from build123d import *

# Parameters (mm, degrees)
SKETCH1_W           = 113
SKETCH1_H           = 53
SKETCH1_R           = 1.25
BOSS_EXTRUDE1_DEPTH = 1.8
SKETCH2_W           = 17
SKETCH2_H           = 12
SKETCH2_W_2         = 8
SKETCH2_H_2         = 14
SKETCH2_W_3         = 18
SKETCH2_H_3         = 10
BOSS_EXTRUDE2_DEPTH = 11


with BuildPart() as part:
    # Sketch1 → Boss-Extrude1 (new body)
    with BuildSketch(Plane.XY):
        with Locations((-56.5, 26.5)):
            Rectangle(SKETCH1_W, SKETCH1_H)
        with Locations((-3, 3)):
            Circle(SKETCH1_R, mode=Mode.SUBTRACT)
        with Locations((-3, 50)):
            Circle(SKETCH1_R, mode=Mode.SUBTRACT)
        with Locations((-105, 50)):
            Circle(SKETCH1_R, mode=Mode.SUBTRACT)
        with Locations((-105, 3)):
            Circle(SKETCH1_R, mode=Mode.SUBTRACT)
    extrude(amount=BOSS_EXTRUDE1_DEPTH)

    # Sketch2 → Boss-Extrude2 (add)
    with BuildSketch(Plane.XY.offset(1.8)):
        with Locations((-9.223845793, 31)):
            Rectangle(SKETCH2_W, SKETCH2_H)
        with Locations((-23.223845793, 42)):
            Rectangle(SKETCH2_W_2, SKETCH2_H_2)
        with Locations((-104, 40)):
            Rectangle(SKETCH2_W_3, SKETCH2_H_3)
        with Locations((-104, 13)):
            Rectangle(SKETCH2_W_3, SKETCH2_H_3)
    extrude(amount=BOSS_EXTRUDE2_DEPTH)


solid = part.part
Geometry check sheet. Reference: the model listing, model coordinates, mm. A direction names the side the tool comes from. Round coordinates to 2 decimals unless told otherwise and drop trailing zeros. Write each loop counter-clockwise with the first axis right and the second up, starting at its lowest first coordinate (ties: lowest second). Pieces come first, ordered by that corner, then holes.
Item 1: Section check D-D (x = -25). Record the boundary of the cut face in (y, z), plus the area to 3 significant figures.
Determined:
outline: (0, 0) - (53, 0) - (53, 1.8) - (49, 1.8) - (49, 12.8) - (35, 12.8) - (35, 1.8) - (0, 1.8) - close
area: 249 mm2
Item 2: Section check C-C (z = 3.25). Record the boundary of the cut face in (x, y), plus the area to 3 significant figures.
Determined:
outline: (-113, 8) - (-95, 8) - (-95, 18) - (-113, 18) - close; (-113, 35) - (-95, 35) - (-95, 45) - (-113, 45) - close; (-27.22, 35) - (-19.22, 35) - (-19.22, 49) - (-27.22, 49) - close; (-17.72, 25) - (-0.72, 25) - (-0.72, 37) - (-17.72, 37) - close
area: 676 mm2
Item 3: Material ranges on line 1 along Y through (x, z) = (-3, 1.1); line 2 along X through (y, z) = (36.5, 7.75); line 3 along Z through (x, y) = (-27.5, 14), recorded low to high.
Determined:
line 1: y = 0 to 1.75, 4.25 to 48.75, 51.25 to 53
line 2: x = -113 to -95, -27.22 to -19.22, -17.72 to -0.72
line 3: z = 0 to 1.8
Item 4: Section check B-B (x = -105). Record the boundary of the cut face in (y, z).
Determined:
outline: (0, 0) - (1.75, 0) - (1.75, 1.8) - (0, 1.8) - close; (4.25, 0) - (48.75, 0) - (48.75, 1.8) - (45, 1.8) - (45, 12.8) - (35, 12.8) - (35, 1.8) - (18, 1.8) - (18, 12.8) - (8, 12.8) - (8, 1.8) - (4.25, 1.8) - close; (51.25, 0) - (53, 0) - (53, 1.8) - (51.25, 1.8) - close
Item 5: Section check A-A (y = 3). Record the boundary of the cut face in (x, z), plus the area to 3 significant figures.
Determined:
outline: (-113, 0) - (-106.25, 0) - (-106.25, 1.8) - (-113, 1.8) - close; (-103.75, 0) - (-4.25, 0) - (-4.25, 1.8) - (-103.75, 1.8) - close; (-1.75, 0) - (0, 0) - (0, 1.8) - (-1.75, 1.8) - close
area: 194 mm2
Item 6: Go/stop test with flat-tipped pins: pin 1 Ø2 at (x, z) = (-93.5, 5.5) entering from +Y; pin 2 Ø3 at (x, y) = (-11.5, 20) entering from -Z; pin 3 Ø3 at (y, z) = (11.5, 10.5) entering from +X; pin 4 Ø2.5 at (x, z) = (-22.5, 7) entering from +Y. Record where each tip stops, or that it passes through.
Determined:
pin 1: passes through
pin 2: stops at z = 0
pin 3: stops at x = -95
pin 4: stops at y = 49
Item 7: Mould release check, pull along X, two halves, no side actions. Record for faces 4 (the face through (-23, 42, 12.8)), 5 (the face through (-95, 13, 7)), 6 (the face through (-103.81, 3.38, 0.89)): +X half, -X half, draft (parallel to the pull), parting line (faces both ways), or undercut.
Determined:
face 4: draft
face 5: +X half
face 6: undercut
Item 8: Access from +Z, -Z, +X, -X, +Y, -Y to the whole of each face (thin tool, end or side, straight path). Record for faces 1 (the face through (-104, 18, 7)), 2 (the face through (-104, 35, 7)), 3 (the face through (-9, 25, 7)).
Determined:
face 1: +Z, +X, -X
face 2: +Z, -X
face 3: +Z, +X, -X, -Y
